Here's how the part is built. I have some questions about the finished solid (model axes, mm). A direction names the side the tool comes from. Coordinates: 2 decimals unless noted, no trailing zeros. Write each loop counter-clockwise with the first axis right and the second up, starting at its lowest first coordinate (ties: lowest second). Pieces come first, ordered by that corner, then holes. Notation, with made-up numbers: (37, 79.5) -> (89, 79.5) arc R15 ccw to (89, 103.5) -> close; hole circle Ø2 at (54, 28). An arc over 180 degrees is marked (long way). Use a Markdown table: item, result. Add a question column.
Item 1: On a 3-axis mill with a long thin cutter (end or side, diameter ignored), from which of +Z, -Z, +X, -X, +Y, -Y can I reach the whole of each face in a straight line? I mean faces 1 (the flat face through (-1, -33, 0)), 2 (the flat face through (0, -25.4, 13)), 3 (the flat face through (45, 50.8, 13)). Say none if no direction works.
Item 2: Imagine slicing it at C-C, the plane z = 12.7. Write out the boundary of the cut face in (x, y) (1 decimal), and give its area (3 significant figures).
Item 3: Imagine slicing it at A-A, the plane y = 63. Count the separate pieces of the cut face and the enclosed holes in it, and give its area (3 significant figures).
Item 4: If we mould it in two halves opening along X, with no side actions, what happens to faces 4 (the flat face through (-44, 50.8, 13)), 5 (the flat face through (-1, -33, 25.4)), 6 (the flat face through (-101.6, -1, 13)), 7 (the cylindrical face through (44.5, -55.63, 12.88))? For each: pulls with the +X half, pulls with the -X half, needs draft (parallel to the pull), parting line crosses it, or undercut.
Item 5: If I drill on line 1 along X through (y, z) = (53.5, 5.75); line 2 along X through (y, z) = (38, 1.5); line 3 along Y through (x, z) = (50.8, 8.5), over which ranges is the centre line in solid material (lowest first)? Write a range as from..to.
Item 6: Imagine slicing it at B-B, the plane y = -50.8. Write out the boundary of the cut face in (x, z), and give its area (3 significant figures).
Item 7: Will this pin go through, and if not, where does the flat tip stop? pin 1 Ø5 at (x, z) = (-15.5, 18.5) entering from +Y.
Item 8: Imagine slicing it at D-D, the plane y = 30. Write out the boundary of the cut face in (x, z).
```python
from build123d import *

# Parameters (mm, degrees)
F0_W     = 203.2
F0_H     = 152.4
F0_R     = 7.9375
F1_DEPTH = 25.4
F2_W     = 50.8
F2_H     = 203.2
F3_DEPTH = 50.8
F4_R     = 7.9375
F5_DEPTH = 25.4
F6_R     = 7.9375
F7_DEPTH = 25.4


with BuildPart() as f1:
    # F0 (on Top) → F1 (new body)
    with BuildSketch(Plane.XY):
        Rectangle(F0_W, F0_H)
        Circle(F0_R, mode=Mode.SUBTRACT)
    extrude(amount=F1_DEPTH)

    # F2 (on face) → F3 (cut)
    with BuildSketch(Plane.XY.offset(25.4)):
        with Locations((0, 76.2)):
            Rectangle(F2_W, F2_H)
    extrude(amount=-F3_DEPTH, mode=Mode.SUBTRACT)

    # F4 (on face) → F5 (cut)
    with BuildSketch(Plane.XY.offset(25.4)):
        with Locations((-50.8, -50.8)):
            Circle(F4_R)
        with Locations((50.8, -50.8)):
            Circle(F4_R)
    extrude(amount=-F5_DEPTH, mode=Mode.SUBTRACT)

    # F6 (on face) → F7 (cut)
    with BuildSketch(Plane(origin=(0, 76.2, 0), x_dir=(-1, 0, 0), z_dir=(0, 1, 0))):
        with Locations((-44.45, 12.7)):
            Circle(F6_R)
        with Locations((44.45, 12.7)):
            Circle(F6_R)
    extrude(amount=-F7_DEPTH, mode=Mode.SUBTRACT)


solid = f1.part
```
Ans:
| question | item | result |
|---|---|---|
| 1 | face 1 | -Z, +X, -X, +Y, -Y |
| 1 | face 2 | +Z, -Z, +Y |
| 1 | face 3 | +Y |
| 2 | outline | (-101.6, -76.2) -> (101.6, -76.2) -> (101.6, 76.2) -> (52.4, 76.2) -> (52.4, 50.8) -> (36.5, 50.8) -> (36.5, 76.2) -> (25.4, 76.2) -> (25.4, -25.4) -> (-25.4, -25.4) -> (-25.4, 76.2) -> (-36.5, 76.2) -> (-36.5, 50.8) -> (-52.4, 50.8) -> (-52.4, 76.2) -> (-101.6, 76.2) -> close; hole circle Ø15.9 at (-50.8, -50.8); hole circle Ø15.9 at (50.8, -50.8) |
| 2 | area | 24,600 mm^2 |
| 3 | separate pieces | 2 |
| 3 | enclosed holes | 2 |
| 3 | area | 3,480 mm^2 |
| 4 | face 4 | undercut |
| 4 | face 5 | needs draft |
| 4 | face 6 | pulls with the -X half |
| 4 | face 7 | undercut |
| 5 | line 1 | x = -101.6..-48.28, -40.62..-25.4, 25.4..40.62, 48.28..101.6 |
| 5 | line 2 | x = -101.6..-25.4, 25.4..101.6 |
| 5 | line 3 | y = -76.2..-58.74, -42.86..50.8 |
| 6 | outline | (-101.6, 0) -> (-58.74, 0) -> (-58.74, 25.4) -> (-101.6, 25.4) -> close; (-42.86, 0) -> (42.86, 0) -> (42.86, 25.4) -> (-42.86, 25.4) -> close; (58.74, 0) -> (101.6, 0) -> (101.6, 25.4) -> (58.74, 25.4) -> close |
| 6 | area | 4,350 mm^2 |
| 7 | pin 1 | stops at y = -25.4 |
| 8 | outline | (-101.6, 0) -> (-25.4, 0) -> (-25.4, 25.4) -> (-101.6, 25.4) -> close; (25.4, 0) -> (101.6, 0) -> (101.6, 25.4) -> (25.4, 25.4) -> close |
